Autodesk Inventor part; units mm, degrees
ref_plane "Anschlussebene-Übergang" through (-40, 13.03, 0) normal (0, 1, 0) x (1, 0, 0)
ref_plane "RWG-X" through (1.8795, 9, 10.525) normal (0, 0, -1) x (-1, 0, 0)
ref_plane "RWG-Y" through (0, 9, 9.585) normal (1, 0, 0) x (0, 0, -1)
sketch "S-Basis" plane through (0, 0, 0) normal (0, 0, 1) x (1, 0, 0)
  line L0 (0, 57.19) -> (0, -57.19) construction
  line L1 (-56, 0) -> (56, 0) construction
  line L2 (1.8795, -0.94) -> (1.8795, 0.94)
  line L3 (1.8795, 0.94) -> (-1.8795, 0.94)
  line L4 (-1.8795, 0.94) -> (-1.8795, -0.94)
  line L5 (-1.8795, -0.94) -> (1.8795, -0.94)
  line L6 (1.8795, -0.94) -> (-1.8795, 0.94) construction
  line L7 (1.8795, 0.94) -> (-1.8795, -0.94) construction
  line L8 (-40, 40.85) -> (40, 40.85)
  line L9 (40, 40.85) -> (40, -40.85)
  line L10 (40, -40.85) -> (-40, -40.85)
  line L11 (-40, -40.85) -> (-40, 40.85)
  line L12 (-40, 40.85) -> (40, -40.85) construction
  line L13 (40, 40.85) -> (-40, -40.85) construction
  line L14 (-40, 33.35) -> (40, 33.35) construction
  circle A0 centre (0, 33.35) radius 2.5 construction
  line L15 (-40, 13.03) -> (40, 13.03) construction
  line L16 (-3.7747, 1.8879) -> (3.7747, 1.8879)
  line L17 (3.7747, 1.8879) -> (3.7747, -1.8879)
  line L18 (3.7747, -1.8879) -> (-3.7747, -1.8879)
  line L19 (-3.7747, -1.8879) -> (-3.7747, 1.8879)
  line L20 (-3.7747, 1.8879) -> (3.7747, -1.8879) construction
  line L21 (3.7747, 1.8879) -> (-3.7747, -1.8879) construction
  circle A1 centre (-32.5, 33.35) radius 2.15
  circle A2 centre (32.5, 33.35) radius 2.15
  circle A3 centre (-32.5, -33.35) radius 2.15
  circle A4 centre (32.5, -33.35) radius 2.15
  line L22 (-3.5, 40.85) -> (3.5, 40.85)
  line L23 (3.5, 40.85) -> (3.5, 27.1517)
  line L24 (3.5, 27.1517) -> (-3.5, 27.1517)
  line L25 (-3.5, 27.1517) -> (-3.5, 40.85)
  point P0 (0, 0)
  point P1 (0, 40.85)
  dimension "d0" = 81.7
  dimension "d1" = 80
  dimension "d2" = 3.759
  dimension "d3" = 1.88
  dimension "d4" = 7.5
  dimension "d5" = 5
  dimension "d6" = 20.32
  dimension "d7" = 4.3
  dimension "d8" = 32.5
  dimension "d9" = 4.3
  dimension "d10" = 32.5
  dimension "d11" = 7.5
  dimension "d23" = 7
ref_plane "Anschlussebene-Übergang" through (-40, 13.03, 0) normal (0, 1, 0) x (1, 0, 0)
extrude "Ex-Base1" add sketch "S-Basis" against normal blind 3 contours L8 L25 L24 L23 L9 L10 L11 | L8 L23 L24 L25 | L16 L17 L18 L19
extrude "Ex-Probe" add sketch "S-Basis" against normal blind 103 contours L16 L17 L18 L19
sketch "Skizze2" plane through (0, 0, 0) normal (1, 0, 0) x (0, 1, 0)
  line L0 (13.03, 14.8668) -> (13.03, -2.4778)
  line L1 (0, 14.8668) -> (0, -2.4778)
  line L2 (-4.8428, 0) -> (16.0088, 0)
  line L3 (13.03, 10.525) -> (9, 10.525)
  line L4 (0, 0) -> (0, 1.525)
  arc A0 (9, 10.525) -> (0, 1.525) centre (9, 1.525) ccw
  dimension "d18" = 10.525
  dimension "d19" = 9
sweep "Sweep-Anschluss" add profiles "S-Basis" path "Skizze2" path curves L4 A0 L3 contours L16 L17 L18 L19
fillet "Rundung1" radius 2 4 edges at (40, -40.85, -1.5) (-40, -40.85, -1.5) (40, 40.85, -1.5) (-40, 40.85, -1.5)
ref_plane "RWG-X" through (1.8795, 9, 10.525) normal (0, 0, -1) x (-1, 0, 0)
ref_plane "RWG-Y" through (0, 9, 9.585) normal (1, 0, 0) x (0, 0, -1)
extrude "Extrusion3" add sketch "S-Basis" along normal blind 6 contours L8 L23 L24 L25
equation "\"d10\" = d8"
equation "\"d11\" = d4"
properties part number "ProbeAntennaDummy"
Verification items for the finished model (mm, model axes). A direction names the side the tool comes from. Round coordinates to 2 decimals unless told otherwise and drop trailing zeros. Loops run counter-clockwise (first coordinate to the right, second up) from the corner with the lowest first, then second, coordinate; pieces in that order, holes last. Notation, with made-up numbers: (5, 82.25) - (47, 82.25) arc R24 ccw to (47, 117.25) - close; hole circle Ø11 at (-35.75, -28.75). An arc over 180 degrees is marked (long way). Use a Markdown table: item, result. Add a question column.
1. Thickness scan on probe 1 along Y at (x, z) = (-32.5, -0.9); probe 2 along Z at (x, y) = (13, 17.5); probe 3 along Y at (x, z) = (-0.5, -68.5). Record the ranges inside material, lowest first. Write a range as [from, to].
2. Gauge pin test, flat ends, axial feed: pin 1 (4 mm diameter, centred on x = -8.5, y = -8, fed in from +Z); pin 2 (2 mm diameter, centred on x = 0.5, y = 31.5, fed in from +Z); pin 3 (4 mm diameter, centred on y = 1, z = -39, fed in from +X); pin 4 (2.5 mm diameter, centred on x = -32.5, y = 33.35, fed in from +Z). Record the tip position at first contact, or that the pin passes through.
3. Section check A-A, the plane x = 32.5. Record the boundary of the cut face in (y, z), plus the area to 3 significant figures.
4. Section check B-B, the plane z = -41.5. Record the boundary of the cut face in (x, y), plus the area to 3 significant figures.
5. Section check C-C, the plane y = 33.35. Record the boundary of the cut face in (x, z), plus the area to 3 significant figures.
6. Release check for a two-part mould opening along Z. For faces 1 (the face through (-1, 40.85, 0)), 2 (the face through (0.05, 1.39, 9.31)), 3 (the face through (1.88, 0, -37)) record: released by +Z, released by -Z, zero draft, split by the parting line, or undercut.
7. Access from +Z, -Z, +X, -X, +Y, -Y to the whole of each face (thin tool, end or side, straight path). Record for faces 4 (the face through (-0.05, 3.92, 6.5)), 5 (the face through (0, -1.888, -52)), 6 (the face through (0, 11, 8.637)), 7 (the face through (0, 11, 9.585)), 8 (the face through (0, -0.94, -50)).
8. Section check D-D, the plane y = -33.35. Record the boundary of the cut face in (x, z), plus the area to 3 significant figures.
Checks:
| question | item | result |
|---|---|---|
| 1 | probe 1 | y = [-40.85, -35.5], [-31.2, 31.2], [35.5, 40.85] |
| 1 | probe 2 | z = [-3, 0] |
| 1 | probe 3 | y = [-1.89, -0.94], [0.94, 1.89] |
| 2 | pin 1 | stops at z = 0 |
| 2 | pin 2 | stops at z = 6 |
| 2 | pin 3 | stops at x = 3.77 |
| 2 | pin 4 | passes through |
| 3 | outline | (-40.85, -3) - (-35.5, -3) - (-35.5, 0) - (-40.85, 0) - close; (-31.2, -3) - (31.2, -3) - (31.2, 0) - (-31.2, 0) - close; (35.5, -3) - (40.85, -3) - (40.85, 0) - (35.5, 0) - close |
| 3 | area | 219 mm^2 |
| 4 | outline | (-3.77, -1.89) - (3.77, -1.89) - (3.77, 1.89) - (-3.77, 1.89) - close; hole (-1.88, -0.94) - (1.88, -0.94) - (1.88, 0.94) - (-1.88, 0.94) - close |
| 4 | area | 21.4 mm^2 |
| 5 | outline | (-40, -3) - (-34.65, -3) - (-34.65, 0) - (-40, 0) - close; (-30.35, -3) - (30.35, -3) - (30.35, 0) - (3.5, 0) - (3.5, 6) - (-3.5, 6) - (-3.5, 0) - (-30.35, 0) - close; (34.65, -3) - (40, -3) - (40, 0) - (34.65, 0) - close |
| 5 | area | 256 mm^2 |
| 6 | face 1 | zero draft |
| 6 | face 2 | released by +Z |
| 6 | face 3 | undercut |
| 7 | face 4 | +X, -X |
| 7 | face 5 | -Z, +X, -X, -Y |
| 7 | face 6 | +X, -X, +Y |
| 7 | face 7 | +Y |
| 7 | face 8 | -Z |
| 8 | outline | (-40, -3) - (-34.65, -3) - (-34.65, 0) - (-40, 0) - close; (-30.35, -3) - (30.35, -3) - (30.35, 0) - (-30.35, 0) - close; (34.65, -3) - (40, -3) - (40, 0) - (34.65, 0) - close |
| 8 | area | 214 mm^2 |
